from build123d import *

# Parameters (mm, degrees)
SKETCH1_R           = 1.6
BOSS_EXTRUDE1_DEPTH = 5
SKETCH3_R           = 11.1
CUT_EXTRUDE1_DEPTH  = 3
SKETCH4_R           = 2.7
CUT_EXTRUDE2_DEPTH  = 3


with BuildPart() as part:
    # Sketch1 → Boss-Extrude1 (new body)
    with BuildSketch(Plane.XY):
        with BuildLine():
            Line((18.357006817, 21.564329359), (-0.634323451, 20.990417665))
            ThreePointArc((-0.634323451, 20.990417665), (-0.95130426, 20.978441796), (-1.268068016, 20.961679406))
            Line((-1.268068016, 20.961679406), (-19.615786314, 20.407217452))
            ThreePointArc((-19.615786314, 20.407217452), (-21.011660375, 19.778980746), (-21.554461954, 18.347718298))
            Line((-21.554461954, 18.347718298), (-21, 0))
            ThreePointArc((-21, 0), (-20.990417665, -0.634323451), (-20.961679406, -1.268068016))
            Line((-20.961679406, -1.268068016), (-20.407217422, -19.615787304))
            ThreePointArc((-20.407217422, -19.615787304), (-19.778980677, -21.011661401), (-18.34771816, -21.55446294))
            Line((-18.34771816, -21.55446294), (0, -21))
            ThreePointArc((0, -21), (0.317197912, -20.99760428), (0.634323451, -20.990417665))
            Line((0.634323451, -20.990417665), (19.62565372, -20.416505971))
            ThreePointArc((19.62565372, -20.416505971), (21.02152778, -19.788269266), (21.564329359, -18.357006817))
            Line((21.564329359, -18.357006817), (20.416505971, 19.62565372))
            ThreePointArc((20.416505971, 19.62565372), (19.788269266, 21.02152778), (18.357006817, 21.564329359))
        make_face()
        with Locations((15.024736206, 15.961118443)):
            Circle(SKETCH1_R, mode=Mode.SUBTRACT)
        with Locations((15.961118443, -15.024736206)):
            Circle(SKETCH1_R, mode=Mode.SUBTRACT)
        with Locations((-15.024736206, -15.961118443)):
            Circle(SKETCH1_R, mode=Mode.SUBTRACT)
        with Locations((-15.961118443, 15.024736206)):
            Circle(SKETCH1_R, mode=Mode.SUBTRACT)
    extrude(amount=BOSS_EXTRUDE1_DEPTH)

    # Sketch3 → Cut-Extrude1 (cut)
    with BuildSketch(Plane.XY.offset(5)):
        Circle(SKETCH3_R)
    extrude(amount=-CUT_EXTRUDE1_DEPTH, mode=Mode.SUBTRACT)

    # Sketch4 → Cut-Extrude2 (cut)
    with BuildSketch(Plane.XY.offset(2)):
        Circle(SKETCH4_R)
    extrude(amount=-CUT_EXTRUDE2_DEPTH, mode=Mode.SUBTRACT)


solid = part.part
For this review, take the finished solid that the model builds, in its own axes (mm). A direction names the side the tool comes from. Round coordinates to 2 decimals unless told otherwise and drop trailing zeros. Loops run counter-clockwise (first coordinate to the right, second up) from the corner with the lowest first, then second, coordinate; pieces in that order, holes last. Notation, with made-up numbers: (89, -20.5) - (135, -20.5) arc R35 cw to (135, 17.5) - close; hole circle Ø2 at (-12.75, -34.75). An arc over 180 degrees is marked (long way). One line per question, with ' | ' between items.
Q1. Tool access review of faces 1 (the cylindrical face through (5.97, 9.36, 3.52)), 2 (the cylindrical face through (13.426, 16.031, 2.465)): name each direction out of +Z, -Z, +X, -X, +Y, -Y from which nothing blocks a thin tool from reaching the whole face with its end or side.
Taken from the geometry:
face 1: +Z | face 2: +Z, -Z
Q2. Take a section at A-A (y = 9). Give the boundary of the cut face in (x, z), and give its area (3 significant figures).
Taken from the geometry:
outline: (-21.27, 0) - (20.74, 0) - (20.74, 5) - (6.5, 5) - (6.5, 2) - (-6.5, 2) - (-6.5, 5) - (-21.27, 5) - close | area: 171 mm²
Q3. The part is to be moulded in two halves that separate along Y. For faces 3 (the flat face through (0, -4, 0)), 4 (the cylindrical face through (-19.79, -21, 2.46)), 5 (the cylindrical face through (19.8, 21.01, 2.46)), 6 (the flat face through (2.3, -2.3, 2)), say which applies: released by +Y, released by -Y, zero draft, split by the parting line, or undercut.
Taken from the geometry:
face 3: zero draft | face 4: released by -Y | face 5: released by +Y | face 6: undercut
Q4. Take a section at C-C (z = 1.1). Give the boundary of the cut face in (x, y).
Taken from the geometry:
outline: (-21.55, 18.35) - (-21, 0) arc R21 ccw to (-20.96, -1.27) - (-20.41, -19.62) arc R2 ccw to (-18.35, -21.55) - (0, -21) arc R21 ccw to (0.63, -20.99) - (19.63, -20.42) arc R2 ccw to (21.56, -18.36) - (20.42, 19.63) arc R2 ccw to (18.36, 21.56) - (-0.63, 20.99) arc R21 ccw to (-1.27, 20.96) - (-19.62, 20.41) arc R2 ccw to start; hole circle Ø3.2 at (-15.96, 15.02); hole circle Ø3.2 at (-15.02, -15.96); hole circle Ø5.4 at (0, 0); hole circle Ø3.2 at (15.02, 15.96); hole circle Ø3.2 at (15.96, -15.02)
Q5. Take a section at B-B (x = -8). Give the boundary of the cut face in (y, z), and give its area (3 significant figures).
Taken from the geometry:
outline: (-21.24, 0) - (20.76, 0) - (20.76, 5) - (7.69, 5) - (7.69, 2) - (-7.69, 2) - (-7.69, 5) - (-21.24, 5) - close | area: 164 mm²
Q6. For line 1 along X through (y, z) = (-16, 0.7); line 2 along X through (y, z) = (16, 1); line 3 along Y through (x, z) = (10, 3.9), list the stretches that pass through material, from the lowest coordinate up. Write a range as [from, to].
Taken from the geometry:
line 1: x = [-20.52, -16.62], [-13.43, 14.69], [17.23, 21.49] | line 2: x = [-21.48, -17.23], [-14.69, 13.43], [16.62, 20.53] | line 3: y = [-20.71, -4.82], [4.82, 21.31]
Q7. Take a section at D-D (x = -12.5). Give the boundary of the cut face in (y, z), and give its area (3 significant figures).
Taken from the geometry:
outline: (-21.38, 0) - (20.62, 0) - (20.62, 5) - (-21.38, 5) - close | area: 210 mm²
Q8. For pin 1 (2.5 mm diameter, centred on x = 15.02, y = 15.96, fed in from -Z); pin 2 (8.5 mm diameter, centred on x = 0, y = 0, fed in from +Z); pin 3 (2 mm diameter, centred on x = 13.5, z = 2.5, fed in from -Y); pin 4 (1.5 mm diameter, centred on y = 5, z = 3.5, fed in from +X), all flat-tipped, find the tip position at first contact; note any pin that passes through.
Taken from the geometry:
pin 1: passes through | pin 2: stops at z = 2 | pin 3: stops at y = -20.63 | pin 4: stops at x = 20.88
